Could you check a few things on this model? Use its own coordinates, in mm. A direction names the side the tool comes from. Give positions to 0.01 mm unless a question says otherwise; leave off trailing zeros. Write each loop counter-clockwise with the first axis right and the second up, starting at its lowest first coordinate (ties: lowest second). Pieces come first, ordered by that corner, then holes. Notation, with made-up numbers: (-8, 62.25) - (11, 62.25) arc R20 ccw to (11, 86.25) - close; hole circle Ø4 at (67.25, -13.75). An arc over 180 degrees is marked (long way). Use one line per item in the form item = value.
```python
from build123d import *

# Parameters (mm, degrees)
SKETCH044_R     = 20
PAD021_DEPTH    = 5
PAD022_DEPTH    = 11
SKETCH051_R     = 1.6
POCKET019_DEPTH = 7.501
SKETCH052_R     = 1.6
POCKET020_DEPTH = 7.501


with BuildPart() as part:
    # Sketch044 (on Face2 of Binder009) → Pad021 (new body)
    with BuildSketch(Plane(origin=(0, 0, 15), x_dir=(-1, 0, 0), z_dir=(0, 0, 1))):
        Circle(SKETCH044_R)
        with BuildLine():
            Line((12.5, 11.521719), (12.5, -11.521719))
            ThreePointArc((-12.5, -11.521719), (0, -17), (12.5, -11.521719))
            Line((-12.5, 11.521719), (-12.5, -11.521719))
            ThreePointArc((12.5, 11.521719), (0, 17), (-12.5, 11.521719))
        make_face(mode=Mode.SUBTRACT)
    extrude(amount=PAD021_DEPTH)

    # Sketch045 (on Face6 of Pad021) → Pad022 (join)
    with BuildSketch(Plane(origin=(0, 0, 15), x_dir=(1, 0, 0), z_dir=(0, 0, -1))):
        with BuildLine():
            ThreePointArc((-14.142136, 14.142136), (-20, 3e-06), (-14.14214, -14.142131))
            Line((-14.14214, -14.142131), (-12.020819, -12.020811))
            ThreePointArc((-12.020815, 12.020815), (-17, 3e-06), (-12.020819, -12.020811))
            Line((-14.142136, 14.142136), (-12.020815, 12.020815))
        make_face()
        with BuildLine():
            ThreePointArc((14.142136, -14.142136), (20, -3e-06), (14.14214, 14.142131))
            Line((14.14214, 14.142131), (12.020819, 12.020811))
            ThreePointArc((12.020815, -12.020815), (17, -3e-06), (12.020819, 12.020811))
            Line((14.142136, -14.142136), (12.020815, -12.020815))
        make_face()
    extrude(amount=PAD022_DEPTH)

    # Sketch051 (on Face2 of Pad021) → Pocket019 (cut, through all)
    with BuildSketch(Plane.YZ.offset(-12.5)):
        with Locations((0, 17.5)):
            Circle(SKETCH051_R)
    extrude(amount=-POCKET019_DEPTH, mode=Mode.SUBTRACT)

    # Sketch052 (on Face12 of Pocket019) → Pocket020 (cut, through all)
    with BuildSketch(Plane(origin=(12.5, 0, 0), x_dir=(0, -1, 0), z_dir=(-1, 0, 0))):
        with Locations((0, 17.5)):
            Circle(SKETCH052_R)
    extrude(amount=-POCKET020_DEPTH, mode=Mode.SUBTRACT)


solid = part.part
```
1. For pin 1 (4 mm diameter, centred on y = -1, z = 14, fed in from -X); pin 2 (4 mm diameter, centred on x = 2.5, z = 16, fed in from +Y); pin 3 (6 mm diameter, centred on y = -12, z = 12, fed in from +X); pin 4 (6.5 mm diameter, centred on x = -6.5, y = 15, fed in from -Z), each with a flat end and sliding along its axis, tell me the tip position at first contact or that it passes through.
Response values:
pin_1 = -20
pin_2 = 19.99
pin_3 = 17.86
pin_4 = 15
2. If I drill on line 1 (Z direction, x = -16, y = 0); line 2 (X direction, y = 0.5, z = 19.5); line 3 (X direction, y = 8.5, z = 17.5), over which ranges is the centre line in solid material (lowest first)? Write a range as from..to.
Response values:
line_1 = 15..15.9, 19.1..20
line_2 = -19.99..-12.5, 12.5..19.99
line_3 = -18.1..-12.5, 12.5..18.1
3. Imagine slicing it at A-A, the plane x = 0. List the corners of the cut face in (y, z) for me.
Response values:
outline = (-20, 15) - (-17, 15) - (-17, 20) - (-20, 20) - close; (17, 15) - (20, 15) - (20, 20) - (17, 20) - close
4. Imagine slicing it at B-B, the plane z = 14.25. List the corners of the cut face in (x, y) for me, and give its area (3 significant figures).
Response values:
outline = (-14.14, -14.14) - (-12.02, -12.02) arc R17 cw to (-12.02, 12.02) - (-14.14, 14.14) arc R20 ccw to start; (12.02, -12.02) - (14.14, -14.14) arc R20 ccw to (14.14, 14.14) - (12.02, 12.02) arc R17 cw to start
area = 174 mm²
5. Which directions (+Z, -Z, +X, -X, +Y, -Y) give clear straight access to the entire face, cutting with the end or side of a thin tool? Please do faces 1 (the face through (17, 0, 10)), 2 (the face through (-13, -13, 10)), 3 (the face through (-13, 13, 10)), 4 (the face through (-12.5, -0.2, 15.2)).
Response values:
face_1 = -Z
face_2 = -Z, -Y
face_3 = -Z, +Y
face_4 = +Z, -Z
6. If we mould it in two halves opening along X, with no side actions, what happens to faces 5 (the face through (-13, 0, 20)), 6 (the face through (12.5, -0.2, 15.2))? For each: pulls with the +X half, pulls with the -X half, needs draft (parallel to the pull), parting line crosses it, or undercut.
Response values:
face_5 = needs draft
face_6 = undercut
7. Imagine slicing it at D-D, the plane y = -13. List the corners of the cut face in (x, z) for me, and give its area (3 significant figures).
Response values:
outline = (-15.2, 4) - (-13, 4) - (-13, 15) - (-10.95, 15) - (-10.95, 20) - (-15.2, 20) - close; (10.95, 15) - (13, 15) - (13, 4) - (15.2, 4) - (15.2, 20) - (10.95, 20) - close
area = 90.8 mm²
8. Imagine slicing it at C-C, the plane y = 0. List the corners of the cut face in (x, z) for me.
Response values:
outline = (-20, 4) - (-17, 4) - (-17, 15) - (-12.5, 15) - (-12.5, 15.9) - (-20, 15.9) - close; (-20, 19.1) - (-12.5, 19.1) - (-12.5, 20) - (-20, 20) - close; (12.5, 15) - (17, 15) - (17, 4) - (20, 4) - (20, 15.9) - (12.5, 15.9) - close; (12.5, 19.1) - (20, 19.1) - (20, 20) - (12.5, 20) - close
